from build123d import *

# Parameters (mm, degrees)
F0_W     = 273.05
F0_H     = 114.3
F0_R     = 38.1
F1_DEPTH = 25.4
F3_DEPTH = 25.4


with BuildPart() as f1:
    # F0 (on Front) → F1 (new body)
    with BuildSketch(Plane.XZ):
        with Locations((136.525, 57.15)):
            Rectangle(F0_W, F0_H)
        with Locations((47.625, 57.15)):
            Circle(F0_R, mode=Mode.SUBTRACT)
        with Locations((225.425, 57.15)):
            Circle(F0_R, mode=Mode.SUBTRACT)
    extrude(amount=F1_DEPTH)

    # F2 (on face) → F3 (cut)
    with BuildSketch(Plane.XZ.offset(25.4)):
        with BuildLine():
            Line((177.8, 114.3), (95.25, 114.3))
            Line((95.25, 114.3), (95.25, 74.93))
            ThreePointArc((95.25, 74.93), (98.597769, 66.847769), (106.68, 63.5))
            Line((106.68, 63.5), (166.37, 63.5))
            ThreePointArc((166.37, 63.5), (174.452231, 66.847769), (177.8, 74.93))
            Line((177.8, 74.93), (177.8, 114.3))
        make_face()
    extrude(amount=-F3_DEPTH, mode=Mode.SUBTRACT)


solid = f1.part
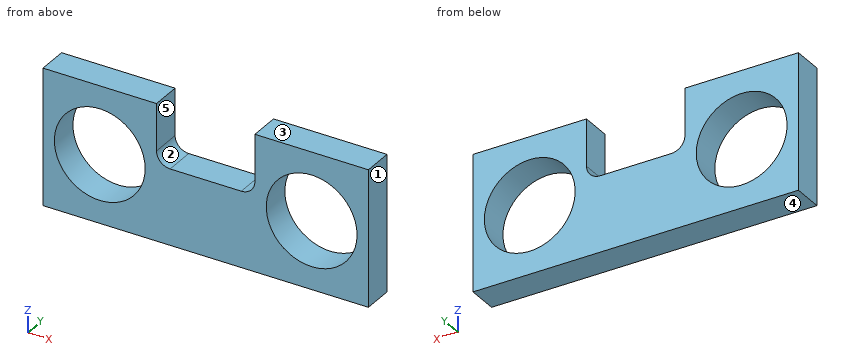
Geometry check sheet. Reference: the model listing, model coordinates, mm. Face numbers are marked on the shaded views. A direction names the side the tool comes from. Round coordinates to 2 decimals unless told otherwise and drop trailing zeros. Loops run counter-clockwise (first coordinate to the right, second up) from the corner with the lowest first, then second, coordinate; pieces in that order, holes last.
Item 1: Cross-section at A-A on y = -9.25. Record the boundary of the cut face in (x, z) (3 decimals), then the cut area to 3 significant figures.
Item 2: Thickness scan on line 1 (X direction, y = -9.25, z = 34); line 2 (X direction, y = -21, z = 103.5); line 3 (X direction, y = -20.5, z = 80.5). Record the ranges inside material, lowest first.
Item 3: Access from +Z, -Z, +X, -X, +Y, -Y to the whole of each face (thin tool, end or side, straight path). Record for the marked faces 4 and 5.
Item 4: Mould release check, pull along X, two halves, no side actions. Record for the marked faces 1, 2 and 3: pulls with the +X half, pulls with the -X half, needs draft (parallel to the pull), parting line crosses it, or undercut.
Item 5: Cross-section at C-C on x = 201.5. Record the boundary of the cut face in (y, z).
Item 6: Cross-section at D-D on x = 132.5. Record the boundary of the cut face in (y, z).
Item 7: Cross-section at B-B on z = 57.15. Record the boundary of the cut face in (x, y) (3 decimals).
Answer sheet:
1. outline: (0, 0) - (273.05, 0) - (273.05, 114.3) - (177.8, 114.3) - (177.8, 74.93) arc R11.43 cw to (166.37, 63.5) - (106.68, 63.5) arc R11.43 cw to (95.25, 74.93) - (95.25, 114.3) - (0, 114.3) - close; hole circle Ø76.2 at (47.625, 57.15); hole circle Ø76.2 at (225.425, 57.15)
1. area: 18,000 mm2
2. line 1: x = 0 to 17.36, 77.89 to 195.16, 255.69 to 273.05
2. line 2: x = 0 to 95.25, 177.8 to 273.05
2. line 3: x = 0 to 17.52, 77.73 to 95.25, 177.8 to 195.32, 255.53 to 273.05
3. face 4: -Z, +X, -X, +Y, -Y
3. face 5: +Z, +Y, -Y
4. face 1: pulls with the +X half
4. face 2: undercut
4. face 3: needs draft
5. outline: (-25.4, 0) - (0, 0) - (0, 27.5) - (-25.4, 27.5) - close; (-25.4, 86.8) - (0, 86.8) - (0, 114.3) - (-25.4, 114.3) - close
6. outline: (-25.4, 0) - (0, 0) - (0, 63.5) - (-25.4, 63.5) - close
7. outline: (0, -25.4) - (9.525, -25.4) - (9.525, 0) - (0, 0) - close; (85.725, -25.4) - (187.325, -25.4) - (187.325, 0) - (85.725, 0) - close; (263.525, -25.4) - (273.05, -25.4) - (273.05, 0) - (263.525, 0) - close
